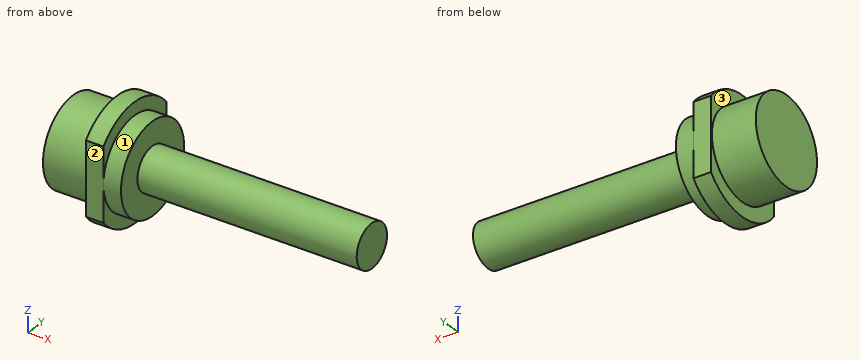
from build123d import *

# Parameters (mm, degrees)
EXTRUDE_1_DEPTH = 2
SKETCH_3_R      = 5.1
EXTRUDE_2_DEPTH = 2
SKETCH_4_R      = 2.45
EXTRUDE_3_DEPTH = 25
SKETCH_5_R      = 4.95
EXTRUDE_4_DEPTH = 5


with BuildPart() as part:
    # 草图2 → 凸台-拉伸1 (new body)
    with BuildSketch(Plane(origin=(0, 0, 0), x_dir=(0, 0, -1), z_dir=(1, 0, 0))):
        with BuildLine():
            Line((4.110048662, 5.1), (-4.110048662, 5.1))
            ThreePointArc((-4.110048662, 5.1), (-6.55, 0), (-4.110048662, -5.1))
            Line((-4.110048662, -5.1), (4.110048662, -5.1))
            ThreePointArc((4.110048662, -5.1), (6.55, 0), (4.110048662, 5.1))
        make_face()
    extrude(amount=EXTRUDE_1_DEPTH)

    # 草图3 → 凸台-拉伸2 (add)
    with BuildSketch(Plane(origin=(2, 0, 0), x_dir=(0, 0, -1), z_dir=(1, 0, 0))):
        Circle(SKETCH_3_R)
    extrude(amount=EXTRUDE_2_DEPTH)

    # 草图4 → 凸台-拉伸3 (add)
    with BuildSketch(Plane(origin=(4, 0, 0), x_dir=(0, 0, -1), z_dir=(1, 0, 0))):
        Circle(SKETCH_4_R)
    extrude(amount=EXTRUDE_3_DEPTH)

    # 草图5 → 凸台-拉伸4 (add)
    with BuildSketch(Plane.ZY):
        Circle(SKETCH_5_R)
    extrude(amount=EXTRUDE_4_DEPTH)


solid = part.part
Could you check a few things on this model? Use its own coordinates, in mm. Face numbers are marked on the shaded views. A direction names the side the tool comes from. Give positions to 0.01 mm unless a question says otherwise; leave off trailing zeros. Write each loop counter-clockwise with the first axis right and the second up, starting at its lowest first coordinate (ties: lowest second). Pieces come first, ordered by that corner, then holes. Notation, with made-up numbers: (62.25, 58.25) -> (82.25, 58.25) arc R32 ccw to (82.25, 92.25) -> close; hole circle Ø9 at (-5, 63). An arc over 180 degrees is marked (long way). Answer as a JSON object with one key per item and string values.
Q1. Please list where these lines run through material, in increasing order: L1, parallel to X at y = 1.75, z = -5.25; L2, parallel to X at y = 4.75, z = -1; L3, parallel to Y at x = -3, z = 0.
Taken from the geometry:
{"L1": "x = 0 to 2", "L2": "x = -5 to 4", "L3": "y = -4.95 to 4.95"}
Q2. Suppose I cut it at D-D on y = -3.5. Write out the boundary of the cut face in (x, z).
Taken from the geometry:
{"outline": "(-5, -3.5) -> (0, -3.5) -> (0, -5.54) -> (2, -5.54) -> (2, -3.71) -> (4, -3.71) -> (4, 3.71) -> (2, 3.71) -> (2, 5.54) -> (0, 5.54) -> (0, 3.5) -> (-5, 3.5) -> close"}
Q3. Will these pins go through, and if not, where does the flat tip stop? pin 1 Ø5 at (y, z) = (0.5, 4) entering from +X; pin 2 Ø1 at (x, z) = (20.5, 4.5) entering from -Y; pin 3 Ø3 at (x, y) = (0.5, -2) entering from -Z; pin 4 Ø4 at (x, z) = (24, -1) entering from +Y.
Taken from the geometry:
{"pin 1": "stops at x = 29", "pin 2": "passes through", "pin 3": "stops at z = -6.53", "pin 4": "stops at y = 2.45"}
Q4. Suppose I cut it at C-C on x = -1. Write out the boundary of the cut face in (y, z), then the cut area to 3 significant figures.
Taken from the geometry:
{"outline": "circle Ø9.9 at (0, 0)", "area": "77.0 mm²"}
Q5. Suppose I cut it at A-A on y = 0. Write out the boundary of the cut face in (x, z).
Taken from the geometry:
{"outline": "(-5, -4.95) -> (0, -4.95) -> (0, -6.55) -> (2, -6.55) -> (2, -5.1) -> (4, -5.1) -> (4, -2.45) -> (29, -2.45) -> (29, 2.45) -> (4, 2.45) -> (4, 5.1) -> (2, 5.1) -> (2, 6.55) -> (0, 6.55) -> (0, 4.95) -> (-5, 4.95) -> close"}
Q6. Which directions (+Z, -Z, +X, -X, +Y, -Y) give clear straight access to the entire face, cutting with the end or side of a thin tool? Please do the marked faces 1, 2 and 3.
Taken from the geometry:
{"face 1": "+X", "face 2": "+Z, -Z, +X, -X, -Y", "face 3": "-X"}
Q7. Suppose I cut it at B-B on z = -1. Write out the boundary of the cut face in (x, y).
Taken from the geometry:
{"outline": "(-5, -4.85) -> (0, -4.85) -> (0, -5.1) -> (2, -5.1) -> (2, -5) -> (4, -5) -> (4, -2.24) -> (29, -2.24) -> (29, 2.24) -> (4, 2.24) -> (4, 5) -> (2, 5) -> (2, 5.1) -> (0, 5.1) -> (0, 4.85) -> (-5, 4.85) -> close"}
